Work out the finished part from the listing and answer in its coordinate system (mm). Round coordinates to 2 decimals unless told otherwise and drop trailing zeros. Loops run counter-clockwise (first coordinate to the right, second up) from the corner with the lowest first, then second, coordinate; pieces in that order, holes last.
```python
from build123d import *

# Parameters (mm, degrees)
SKETCH_2_R      = 2.6
SKETCH_2_R_2    = 5
EXTRUDE_1_DEPTH = 4


with BuildPart() as part:
    # 草图2 → 凸台-拉伸1 (new body)
    with BuildSketch(Plane.XY):
        with BuildLine():
            Line((17.886574367, 34.937240644), (80.386574367, 8.968504219))
            ThreePointArc((80.386574367, 8.968504219), (90.386574367, -1.031495781), (80.386574367, -11.031495781))
            Line((80.386574367, -11.031495781), (17.886574367, -37.000232206))
            ThreePointArc((17.886574367, -37.000232206), (-39.613425633, -1.031495781), (17.886574367, 34.937240644))
        make_face()
        with Locations((0.386574367, -24.781495781)):
            Circle(SKETCH_2_R, mode=Mode.SUBTRACT)
        with Locations((19.872145952, -12.281495781)):
            Circle(SKETCH_2_R, mode=Mode.SUBTRACT)
        with Locations((0.386574367, -1.031495781)):
            Circle(SKETCH_2_R_2, mode=Mode.SUBTRACT)
        with Locations((-20.181528973, 10.843504219)):
            Circle(SKETCH_2_R, mode=Mode.SUBTRACT)
        with Locations((20.954677707, 10.843504219)):
            Circle(SKETCH_2_R, mode=Mode.SUBTRACT)
        with Locations((-19.098997218, -12.281495781)):
            Circle(SKETCH_2_R, mode=Mode.SUBTRACT)
        with Locations((0.386574367, 21.468504219)):
            Circle(SKETCH_2_R, mode=Mode.SUBTRACT)
        with Locations((80.386574367, -1.031495781)):
            Circle(SKETCH_2_R_2, mode=Mode.SUBTRACT)
    extrude(amount=EXTRUDE_1_DEPTH)


solid = part.part
```
1. Given pin 1 (7 mm diameter, centred on x = -19.1, y = -12.28, fed in from +Z), flat-ended and moving along its own axis, determine where the tip first touches the part or whether it passes through.
Answer key:
pin 1: stops at z = 4
2. Find section C-C (x = 39.5). Write down the section's boundary in (y, z), then the cut area to 3 significant figures.
Answer key:
outline: (-28.02, 0) - (25.96, 0) - (25.96, 4) - (-28.02, 4) - close
area: 216 mm2
3. Determine the mould class of faces 1 (the face through (19.31, -14.82, 1.97)), 2 (the face through (-39.597, -2.165, 1.972)), 3 (the face through (0.048, 24.046, 1.972)), 4 (the face through (12, 0, 4)) for opening direction Y: +Y half, -Y half, draft (parallel to the pull), parting line (faces both ways), or undercut.
Answer key:
face 1: undercut
face 2: parting line
face 3: undercut
face 4: draft
4. Find section A-A (z = 2.3). Give the number of separate pieces and of enclosed holes in the cut face, then the cut area to 3 significant figures.
Answer key:
separate pieces: 1
enclosed holes: 8
area: 6,610 mm2
5. Find section B-B (y = 15). Write down the section's boundary in (x, z), then the cut area to 3 significant figures.
Answer key:
outline: (-36.26, 0) - (65.87, 0) - (65.87, 4) - (-36.26, 4) - close
area: 409 mm2
6. Consider probe 1 along Y at (x, z) = (20.5, 2.8); probe 2 along X at (y, z) = (12.5, 3.35); probe 3 along X at (y, z) = (10.5, 1.3). Determine where each line is inside the solid, lowest interval first.
Answer key:
probe 1: y = -35.91 to -14.8, -9.76 to 8.28, 13.4 to 33.85
probe 2: x = -37.26 to -22.19, -18.18 to 18.95, 22.96 to 71.89
probe 3: x = -37.92 to -22.76, -17.6 to 18.38, 23.53 to 76.7
